Build history of the part. All positions in model axes, mm. Coordinates: 2 decimals unless noted, no trailing zeros. Loops run counter-clockwise (first coordinate to the right, second up) from the corner with the lowest first, then second, coordinate; pieces in that order, holes last. Notation, with made-up numbers: (-26.75, 36) -> (14.25, 36) arc R20 ccw to (14.25, 73) -> close; hole circle Ø10 at (83.5, 11). An arc over 180 degrees is marked (long way). One line per item, written item: value. Start each with the question number.
```python
from build123d import *

# Parameters (mm, degrees)
SKETCH1_W           = 241.3
SKETCH1_H           = 114.3
SKETCH1_R           = 12.7
SKETCH1_R_2         = 3.175
BOSS_EXTRUDE1_DEPTH = 6.35


with BuildPart() as part:
    # Sketch1 → Boss-Extrude1 (new body)
    with BuildSketch(Plane(origin=(0, 0, 0), x_dir=(1, 0, 0), z_dir=(0, 1, 0))):
        with Locations((120.65, 57.15)):
            Rectangle(SKETCH1_W, SKETCH1_H)
        with Locations((38.1, 57.15)):
            Circle(SKETCH1_R, mode=Mode.SUBTRACT)
        with Locations((88.9, 104.775)):
            Circle(SKETCH1_R_2, mode=Mode.SUBTRACT)
        with Locations((139.7, 104.775)):
            Circle(SKETCH1_R_2, mode=Mode.SUBTRACT)
        with Locations((139.7, 9.525)):
            Circle(SKETCH1_R_2, mode=Mode.SUBTRACT)
        with Locations((88.9, 9.525)):
            Circle(SKETCH1_R_2, mode=Mode.SUBTRACT)
        with Locations((18.983968606, 76.2)):
            Circle(SKETCH1_R_2, mode=Mode.SUBTRACT)
        with Locations((18.983968606, 38.1)):
            Circle(SKETCH1_R_2, mode=Mode.SUBTRACT)
        with Locations((57.216031394, 38.1)):
            Circle(SKETCH1_R_2, mode=Mode.SUBTRACT)
        with Locations((57.216031394, 76.2)):
            Circle(SKETCH1_R_2, mode=Mode.SUBTRACT)
        with BuildLine():
            ThreePointArc((188.131704345, 68.331953125), (190.5, 45.72), (192.868295655, 68.331953125))
            ThreePointArc((192.868295655, 68.331953125), (190.5, 70.96125), (188.131704345, 68.331953125))
        make_face(mode=Mode.SUBTRACT)
    extrude(amount=BOSS_EXTRUDE1_DEPTH)


solid = part.part
```
Item 1: Band-saw the part on A-A, the plane x = 88.9. List the corners of the cut face in (y, z).
Item 2: Band-saw the part on D-D, the plane y = 4.25. Count the separate pieces of the cut face and the enclosed holes in it, and give its area (3 significant figures).
Item 3: Band-saw the part on B-B, the plane x = 38.1. List the corners of the cut face in (y, z).
Item 4: Drop a flat-ended pin along its axis: pin 1 Ø7.5 at (x, z) = (139.7, -9.525) entering from -Y. Give the stop position or say it passes through.
Item 5: Two-plate mould, pull along Z, no slides. Class faces 1 (the face through (43.96, 3.131, -45.883)), 2 (the face through (119, 3, -114.3)), 3 (the face through (119, 3, 0)), 4 (the face through (119, 6.35, -58)): +Z half, -Z half, draft (parallel to the pull), parting line (faces both ways), or undercut.
Item 6: Probe probe 1 along Z at (x, y) = (139.7, 4.25); probe 2 along X at (y, z) = (3.5, -38.1); probe 3 along X at (y, z) = (4.5, -36). List the from-to ranges inside material, lowest first.
Item 7: Band-saw the part on C-C, the plane z = -38.1. List the corners of the cut face in (x, y).
Worked out:
1. outline: (0, -114.3) -> (6.35, -114.3) -> (6.35, -107.95) -> (0, -107.95) -> close; (0, -101.6) -> (6.35, -101.6) -> (6.35, -12.7) -> (0, -12.7) -> close; (0, -6.35) -> (6.35, -6.35) -> (6.35, 0) -> (0, 0) -> close
2. separate pieces: 1
2. enclosed holes: 10
2. area: 26,400 mm²
3. outline: (0, -114.3) -> (6.35, -114.3) -> (6.35, -69.85) -> (0, -69.85) -> close; (0, -44.45) -> (6.35, -44.45) -> (6.35, 0) -> (0, 0) -> close
4. pin 1: stops at y = 0
5. face 1: undercut
5. face 2: -Z half
5. face 3: +Z half
5. face 4: draft
6. probe 1: z = -114.3 to -107.95, -101.6 to -12.7, -6.35 to 0
6. probe 2: x = 0 to 15.81, 22.16 to 54.04, 60.39 to 241.3
6. probe 3: x = 0 to 16.6, 21.37 to 54.83, 59.6 to 241.3
7. outline: (0, 0) -> (15.81, 0) -> (15.81, 6.35) -> (0, 6.35) -> close; (22.16, 0) -> (54.04, 0) -> (54.04, 6.35) -> (22.16, 6.35) -> close; (60.39, 0) -> (241.3, 0) -> (241.3, 6.35) -> (60.39, 6.35) -> close
